Autodesk Inventor part; units mm, degrees
ref_plane "YZ Plane" through (0, 0, 0) normal (1, 0, 0) x (0, 1, 0)
ref_plane "XZ Plane" through (0, 0, 0) normal (0, 1, 0) x (-1, 0, 0)
ref_plane "XY Plane" through (0, 0, 0) normal (0, 0, 1) x (1, 0, 0)
sketch "Sketch1" plane through (0, 0, 0) normal (0, 0, 1) x (1, 0, 0)
  circle A0 centre (0, 0) radius 50
  point P0 (0, 44.5)
extrude "Extrusion1" add sketch "Sketch1" along normal blind 10
sketch "Sketch4" plane through (0, 0, 10) normal (0, 0, 1) x (1, 0, 0)
  circle A0 centre (0, 0) radius 40
  circle A1 centre (0, 0) radius 50
  dimension "d20" = 80
extrude "Extrusion4" add sketch "Sketch4" along normal blind 23
hole "Hole2" at (0, 44.5, 0) direction (0, 0, 1) diameter 4.134 end through all counterbore diameter 7 counterbore depth 2
pattern_circular "Circular Pattern2" count 8 over 360 about axis through (0, 0, -10) along (0, 0, 1) of "Hole2"
sketch "Sketch5" plane through (0, 0, 0) normal (0, 0, -1) x (-1, 0, 0)
  circle A0 centre (0, 0) radius 7.5
  dimension "d34" = 15
extrude "Extrusion5" cut sketch "Sketch5" against normal through all
sketch "Sketch6" plane through (0, 0, 0) normal (0, 0, -1) x (-1, 0, 0)
  circle A0 centre (0, 0) radius 7.5
  circle A1 centre (0, 0) radius 50
sketch "Sketch8" plane through (0, 0, 10) normal (0, 0, 1) x (1, 0, 0)
  circle A0 centre (0, 0) radius 12.5
  circle A1 centre (0, 0) radius 7.5
  dimension "d50" = 25
extrude "Extrusion7" add sketch "Sketch8" along normal blind 20
chamfer "Chamfer1" distance 2 angle 45 2 edges at (-7.5, 0, 30) (-12.5, 0, 30)
fillet "Fillet1" radius 2 2 edges at (-12.5, 0, 10) (-40, 0, 10)
chamfer "Chamfer2" distance 2 angle 45 1 edges at (7.5, 0, 0)
properties part number "Cycloidal gear cover front"
Geometry check sheet. Reference: the model listing, model coordinates, mm. A direction names the side the tool comes from. Give positions to 0.01 mm unless a question says otherwise; leave off trailing zeros. Write each loop counter-clockwise with the first axis right and the second up, starting at its lowest first coordinate (ties: lowest second). Pieces come first, ordered by that corner, then holes. Notation, with made-up numbers: (39.25, 52) - (94.25, 52) arc R16 cw to (94.25, 73) - close; hole circle Ø7 at (-11.75, -5.5). An arc over 180 degrees is marked (long way). Use a Markdown table: item, result.
Q1. Section check B-B, the plane x = 44.5. Enter the section's corners in (y, z), then the cut area to 3 significant figures.
Computed:
| item | result |
|---|---|
| outline | (-22.8, 0) - (-3.5, 0) - (-3.5, 2) - (-2.07, 2) - (-2.07, 33) - (-22.8, 33) - close; (2.07, 2) - (3.5, 2) - (3.5, 0) - (22.8, 0) - (22.8, 33) - (2.07, 33) - close |
| area | 1,360 mm² |
Q2. Go/stop test with flat-tipped pins: P1, Ø12, axis at y = 22, z = 21.5, coming from the +X side; P2, Ø3, axis at x = 32, z = 21.5, coming from the -Y side; P3, Ø12, axis at x = 5, z = 23, coming from the +Y side; P4, Ø3.5, axis at x = 31.47, y = 31.47, coming from the +Z side. Record where each tip stops, or that it passes through.
Computed:
| item | result |
|---|---|
| P1 | stops at x = 47.37 |
| P2 | stops at y = -39.62 |
| P3 | stops at y = 50 |
| P4 | passes through |
Q3. Draft check along Y on faces 1 (the face through (47.69, -15.02, 16.27)), 2 (the face through (-15, 37.3, 33)), 3 (the face through (32.73, -29.83, 17.72)). Enter one of: pulls with the +Y half, pulls with the -Y half, needs draft (parallel to the pull), parting line crosses it, or undercut.
Computed:
| item | result |
|---|---|
| face 1 | parting line crosses it |
| face 2 | needs draft |
| face 3 | undercut |
Q4. Thickness scan on L1, parallel to X at y = 32, z = 31; L2, parallel to Z at x = 4, y = 15; L3, parallel to Y at x = 45, z = 20.5. Record the ranges inside material, lowest first. Write a range as [from, to].
Computed:
| item | result |
|---|---|
| L1 | x = [-38.42, -33.46], [-29.47, -24], [24, 29.47], [33.46, 38.42] |
| L2 | z = [0, 10] |
| L3 | y = [-21.79, -2.01], [2.01, 21.79] |
Q5. Section check A-A, the plane z = 14. Give the number of separate pieces and of enclosed holes in the cut face, then the cut area to 3 significant figures.
Computed:
| item | result |
|---|---|
| separate pieces | 2 |
| enclosed holes | 10 |
| area | 3,030 mm² |
Q6. Set-up check for faces 4 (the face through (-29.83, -32.73, 17.72)), 5 (the face through (-33.6, 28.69, 1.01)), 6 (the face through (-1, -16, 10)): record each of +Z, -Z, +X, -X, +Y, -Y from which the full face is reachable in a straight line by a thin tool's end or side.
Computed:
| item | result |
|---|---|
| face 4 | +Z, -Z |
| face 5 | -Z |
| face 6 | +Z |
